Read the model definition and answer for the solid it produces. Units are mm, in the model's axes. A direction names the side the tool comes from. Coordinates: 2 decimals unless noted, no trailing zeros. Order: outer loops, then holes, each group sorted by start corner. A loop starts at its lowest first (then second) coordinate and runs counter-clockwise, first axis right, second up.
from build123d import *

# Parameters (mm, degrees)
BOSS_EXTRUDE1_DEPTH = 2.4
FILLET1_R           = 2


with BuildPart() as part:
    # Sketch1 → Boss-Extrude1 (new body)
    with BuildSketch(Plane(origin=(0, 0, 0), x_dir=(1, 0, 0), z_dir=(0, 1, 0))):
        Polygon((27.8, 2.1), (27.8, 0), (33.3, 0), (33.3, 15.15), (27.8, 15.15), (27.8, 13.05), (0, 13.05), (0, 2.1), align=None)
        with BuildLine():
            ThreePointArc((4.45, 5.875), (2.75, 7.575), (4.45, 9.275))
            Line((4.45, 9.275), (6.25, 9.275))
            ThreePointArc((6.25, 9.275), (7.95, 7.575), (6.25, 5.875))
            Line((6.25, 5.875), (4.45, 5.875))
        make_face(mode=Mode.SUBTRACT)
        with BuildLine():
            ThreePointArc((23.1, 9.275), (24.8, 7.575), (23.1, 5.875))
            Line((23.1, 5.875), (21.3, 5.875))
            ThreePointArc((21.3, 5.875), (19.6, 7.575), (21.3, 9.275))
            Line((21.3, 9.275), (23.1, 9.275))
        make_face(mode=Mode.SUBTRACT)
    extrude(amount=-BOSS_EXTRUDE1_DEPTH)

    # Fillet1
    fillet1_edges = [part.edges().sort_by_distance(p)[0] for p in [
        (33.3, -1.2, -15.15),
        (33.3, -1.2, 0),
        (0, -1.2, -2.1),
        (0, -1.2, -13.05),
    ]]
    fillet(fillet1_edges, radius=FILLET1_R)


solid = part.part
Q1. Each of these flat-tipped pins is pushed along its axis until it touches: P1, Ø4, axis at x = 12, z = -5.5, coming from the +Y side; P2, Ø0.5, axis at x = 22.5, y = -1, coming from the -Z side; P3, Ø0.6, axis at y = -0.5, z = -1.5, coming from the -X side; P4, Ø0.5, axis at x = 5.5, y = -1, coming from the +Z side. Where does it stop, or does it pass through?
Q2. The part is cut by section A-A, the plane y = -1.15. Determine the outline of the cut face in (x, z) (3 decimals).
Q3. Straight lines are drawn through the part: L1, parallel to X at y = -1.25, z = -9; L2, parallel to Z at x = 14, y = -1.5; L3, parallel to Z at x = 24, y = -1. For each, find the intervals that lie inside material, in ascending order.
Q4. The part is cut by section B-B, the plane z = -7.25. Determine the outline of the cut face in (x, y), then the cut area to 3 significant figures.
Q5. Which of the six approach directions +Z, -Z, +X, -X, +Y, -Y give full straight-line access (tool end or side, diameter ignored) to faces 1 (the flat face through (15, -1, -2.1)), 2 (the flat face through (5, -1, -9.275)), 3 (the flat face through (27.8, -1, -14)), 4 (the flat face through (16, -2.4, -8))?
Q6. The part is cut by section D-D, the plane z = -13.5. Determine the outline of the cut face in (x, y), then the cut area to 3 significant figures.
Q7. The part is cut by section C-C, the plane x = 26. Determine the outline of the cut face in (y, z).
Q8. Determine the mould class of faces 5 (the flat face through (30, -1, -15.15)), 6 (the flat face through (5, -1, -5.875)), 7 (the cylindrical face through (32.73, -1.22, -14.55)) for opening direction X: +X half, -X half, draft (parallel to the pull), parting line (faces both ways), or undercut.
Computed values:
1. P1: stops at y = 0
1. P2: stops at z = -13.05
1. P3: stops at x = 27.8
1. P4: stops at z = -2.1
2. outline: (0, -11.05) arc R2 ccw to (2, -13.05) - (27.8, -13.05) - (27.8, -15.15) - (31.3, -15.15) arc R2 ccw to (33.3, -13.15) - (33.3, -2) arc R2 ccw to (31.3, 0) - (27.8, 0) - (27.8, -2.1) - (2, -2.1) arc R2 ccw to (0, -4.1) - close; hole (4.45, -9.275) - (6.25, -9.275) arc R1.7 ccw to (6.25, -5.875) - (4.45, -5.875) arc R1.7 ccw to start; hole (21.3, -9.275) - (23.1, -9.275) arc R1.7 ccw to (23.1, -5.875) - (21.3, -5.875) arc R1.7 ccw to start
3. L1: x = 0 to 3.52, 7.18 to 20.37, 24.03 to 33.3
3. L2: z = -13.05 to -2.1
3. L3: z = -13.05 to -9.02, -6.13 to -2.1
4. outline: (0, -2.4) - (2.78, -2.4) - (2.78, 0) - (0, 0) - close; (7.92, -2.4) - (19.63, -2.4) - (19.63, 0) - (7.92, 0) - close; (24.77, -2.4) - (33.3, -2.4) - (33.3, 0) - (24.77, 0) - close
4. area: 55.3 mm2
5. face 1: +Z, -X, +Y, -Y
5. face 2: +Y, -Y
5. face 3: -Z, -X, +Y, -Y
5. face 4: +Z, -Z, +X, -X, -Y
6. outline: (27.8, -2.4) - (33.27, -2.4) - (33.27, 0) - (27.8, 0) - close
6. area: 13.1 mm2
7. outline: (-2.4, -13.05) - (0, -13.05) - (0, -2.1) - (-2.4, -2.1) - close
8. face 5: draft
8. face 6: undercut
8. face 7: +X half
